Geometry check sheet. Reference: the model listing, model coordinates, mm. Face numbers are marked on the shaded views. A direction names the side the tool comes from. Give positions to 0.01 mm unless a question says otherwise; leave off trailing zeros. Order: outer loops, then holes, each group sorted by start corner. A loop starts at its lowest first (then second) coordinate and runs counter-clockwise, first axis right, second up. Notation, with made-up numbers: (39, 38.25) - (81, 38.25) arc R21 cw to (81, 53.25) - close; hole circle Ø11 at (73, 56.5). An arc over 180 degrees is marked (long way). Put each result on its own line as item: value. Start each with the question number.
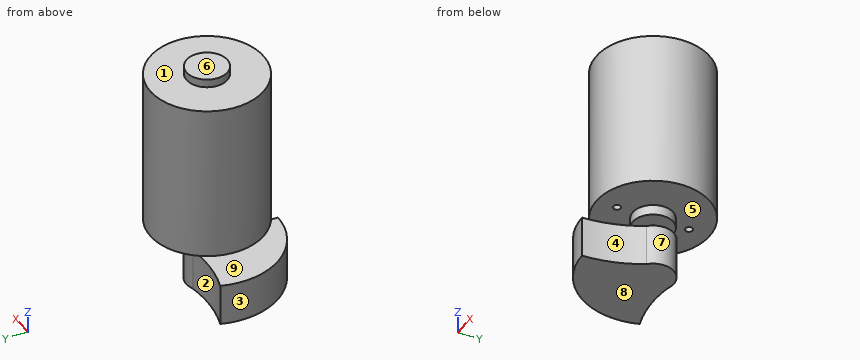
Autodesk Inventor part; units mm, degrees
ref_plane "YZ Plane" through (0, 0, 0) normal (1, 0, 0) x (0, 1, 0)
ref_plane "XZ Plane" through (0, 0, 0) normal (0, 1, 0) x (-1, 0, 0)
ref_plane "XY Plane" through (0, 0, 0) normal (0, 0, 1) x (1, 0, 0)
sketch "スケッチ1" plane through (0, 0, 0) normal (0, 0, 1) x (1, 0, 0)
  circle A0 centre (0, 0) radius 13.6
  dimension "d0" = 27.2
extrude "押し出し1" add sketch "スケッチ1" along normal mid plane 38
sketch "スケッチ2" plane through (0, 0, 19) normal (0, 0, 1) x (1, 0, 0)
  circle A0 centre (0, 0) radius 4.9
  dimension "d3" = 9.8
extrude "押し出し2" add sketch "スケッチ2" along normal blind 2
sketch "スケッチ3" plane through (0, 0, -19) normal (0, 0, -1) x (-1, 0, 0)
  circle A0 centre (0, 0) radius 4.85
  dimension "d6" = 9.7
extrude "押し出し3" add sketch "スケッチ3" along normal blind 2.5
sketch "スケッチ4" plane through (0, 0, -21.5) normal (0, 0, -1) x (-1, 0, 0)
  circle A0 centre (0, 0) radius 4.85
  circle A1 centre (0, 0) radius 1
  dimension "d9" = 2
extrude "押し出し4" add sketch "スケッチ4" along normal blind 3 contours A1
sketch "スケッチ5" plane through (0, 0, -24.5) normal (0, 0, -1) x (-1, 0, 0)
  circle A0 centre (0, 0) radius 5
  circle A1 centre (0, 0) radius 1
  circle A2 centre (0, 0) radius 17
  line L0 (0, 0) -> (0, -17)
  line L1 (0, 0) -> (16.168, 5.2533)
  circle A3 centre (0, 0) radius 4.85
  line L2 (0, 0) -> (-4.7553, -1.5451)
  line L3 (0, 0) -> (0, 5)
  arc A4 (0, -17) -> (-4.7553, -1.5451) centre (-29.9902, -17.7686) ccw
  arc A5 (0, 5) -> (16.168, 5.2533) centre (7.6314, 34.0131) ccw
  point P0 (2.1361, 4.5207)
  point P1 (-3.6394, -3.4286)
  dimension "d12" = 10
  dimension "d13" = 34
  dimension "d14" = 108
  dimension "d15" = 108
  dimension "d16" = 72
  dimension "d17" = 30
  dimension "d18" = 30
extrude "押し出し5" add sketch "スケッチ5" along normal blind 10 contours L3 A3 L2 A0 | A5 A0 L1 A3 L3 | A0 A5 | A4 A0 | L2 A3 L0 A0 A4 | A5 L1 A0 | L3 A1 L2 A3 | A3 L1 A1 L3 | A0 L0 A4 | L2 A1 L0 A3 | L1 A2 L0 A0 | A0 L0 A3 L1 | A3 L0 A1 L1 | L3 L2 A1 | A1 L1 L3 | L2 L0 A1 | A1 L0 L1
sketch "スケッチ6" plane through (0, 0, -19) normal (0, 0, -1) x (-1, 0, 0)
  circle A0 centre (0, 0) radius 4.85
  circle A1 centre (0, 0) radius 13.6
  point P0 (0, 8.6)
  point P1 (0, -8.6)
  dimension "d21" = 8.6
  dimension "d22" = 8.6
hole "穴1" at (0, 8.6, -19) at (0, -8.6, -19) direction (0, 0, 1) diameter 1.7294 depth 5.5 tip angle 118
equation "\"d15\" = d14"
properties part number "Vibration_motor"
Item 1: Release check for a two-part mould opening along Z. For the marked faces 6, 7, 8 and 9 record: +Z half, -Z half, draft (parallel to the pull), parting line (faces both ways), or undercut.
Item 2: Thickness scan on line 1 along Z through (x, y) = (-10.5, -4); line 2 along Y through (x, z) = (0, -16.05); line 3 along Y through (x, z) = (0.5, -18.5). Record the ranges inside material, lowest first.
Item 3: Cross-section at D-D (z = -23). Enter the section's corners in (x, y).
Item 4: Cross-section at B-B (x = -5.5). Enter the section's corners in (y, z), and give its area (3 significant figures).
Item 5: Cross-section at C-C (z = 0.5). Enter the section's corners in (x, y), and give its area (3 significant figures).
Item 6: Set-up check for the marked faces 1, 2, 3, 4 and 5: record each of +Z, -Z, +X, -X, +Y, -Y from which the full face is reachable in a straight line by a thin tool's end or side.
Item 7: Gauge pin test, flat ends, axial feed: pin 1 Ø8 at (y, z) = (-3.5, -16.5) entering from +X; pin 2 Ø1.6 at (x, y) = (0, 8.6) entering from +Z; pin 3 Ø12 at (x, z) = (-1.5, 8) entering from -Y; pin 4 Ø4 at (y, z) = (-11, 2.5) entering from -X. Record the tip position at first contact, or that the pin passes through.
Item 8: Cross-section at A-A (y = 0). Enter the section's corners in (x, z), and give its area (3 significant figures).
Recorded:
1. face 6: +Z half
1. face 7: draft
1. face 8: -Z half
1. face 9: undercut
2. line 1: z = -34.5 to -24.5, -19 to 19
2. line 2: y = -13.6 to -9.46, -7.74 to 7.74, 9.46 to 13.6
2. line 3: y = -13.59 to -9.31, -7.89 to 7.89, 9.31 to 13.59
3. outline: circle Ø2 at (0, 0)
4. outline: (-16.09, -34.5) - (4.09, -34.5) - (4.09, -24.5) - (-16.09, -24.5) - close; (-12.44, -19) - (12.44, -19) - (12.44, 19) - (-12.44, 19) - close
4. area: 1,150 mm^2
5. outline: circle Ø27.2 at (0, 0)
5. area: 581 mm^2
6. face 1: +Z
6. face 2: -Z, +Y
6. face 3: +Z, -Z, -X
6. face 4: -Z, +X, -Y
6. face 5: none
7. pin 1: stops at x = 13.6
7. pin 2: stops at z = 19
7. pin 3: stops at y = -13.6
7. pin 4: stops at x = -10.2
8. outline: (-17, -34.5) - (5, -34.5) - (5, -24.5) - (1, -24.5) - (1, -21.5) - (4.85, -21.5) - (4.85, -19) - (13.6, -19) - (13.6, 19) - (4.9, 19) - (4.9, 21) - (-4.9, 21) - (-4.9, 19) - (-13.6, 19) - (-13.6, -19) - (-4.85, -19) - (-4.85, -21.5) - (-1, -21.5) - (-1, -24.5) - (-17, -24.5) - close
8. area: 1,300 mm^2
